from build123d import *

# Parameters (mm, degrees)
BOSS_EXTRUDE1_DEPTH      = 63.25
BOSS_EXTRUDE1_DEPTH_BACK = 63.25
CHAMFER1_SIZE            = 0.21


with BuildPart() as part:
    # Sketch3 → Boss-Extrude1 (new, two sides: drawn at the far end of the back side and taken through both)
    with BuildSketch(Plane.XY.offset(-BOSS_EXTRUDE1_DEPTH_BACK)):
        with BuildLine():
            Line((-2.5, 3.538348415), (-2.5, 6.538348415))
            ThreePointArc((-2.5, 6.538348415), (0, -7), (2.5, 6.538348415))
            Line((2.5, 6.538348415), (2.5, 3.538348415))
            Line((2.5, 3.538348415), (-2.5, 3.538348415))
        make_face()
    extrude(amount=BOSS_EXTRUDE1_DEPTH + BOSS_EXTRUDE1_DEPTH_BACK)

    # Chamfer1
    chamfer1_edges = [part.edges().sort_by_distance(p)[0] for p in [
        (0, -7, -63.25),
        (0, -7, 63.25),
    ]]
    chamfer(chamfer1_edges, length=CHAMFER1_SIZE)


solid = part.part
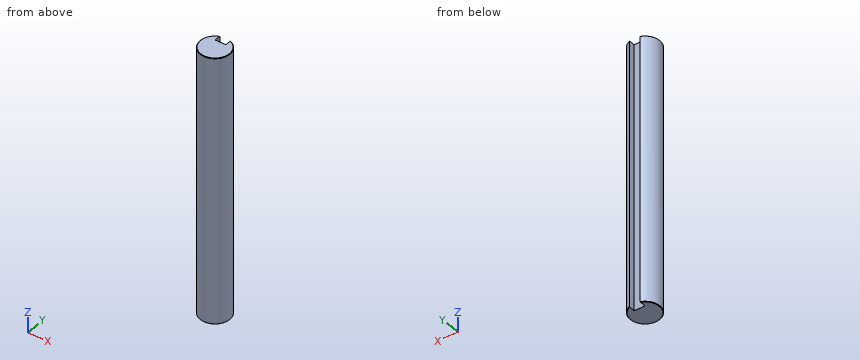
Could you check a few things on this model? Use its own coordinates, in mm. Give positions to 0.01 mm unless a question says otherwise; leave off trailing zeros. Write each loop counter-clockwise with the first axis right and the second up, starting at its lowest first coordinate (ties: lowest second). Pieces come first, ordered by that corner, then holes. Notation, with made-up numbers: (14, 80) -> (59, 80) arc R21 cw to (59, 113) -> close; hole circle Ø1 at (-32, 40). An arc over 180 degrees is marked (long way). Answer as CSV lines item,"result". Start each with the question number.
(1) If we section it at B-B, the plane x = 0: Write out the boundary of the cut face in (y, z), and give its area (3 significant figures).
(2) If we section it at A-A, the plane z = -0.5: Write out the boundary of the cut face in (x, y).
(3) Please list where these lines run through material, in increasing order: line 1 (X direction, y = 5.25, z = 34); line 2 (X direction, y = 4.25, z = 42); line 3 (Y direction, x = -0.25, z = 56).
(4) I'm going to push flat-ended pins straight in: pin 1 Ø2 at (x, z) = (4.5, -39) entering from -Y; pin 2 Ø0.9 at (y, z) = (4.5, 28) entering from -X; pin 3 Ø5 at (x, z) = (4.5, 29.5) entering from -Y. Where does each tip first touch, or does it pass through?
Answer list:
1,outline,"(-7, -63.04) -> (-6.79, -63.25) -> (3.54, -63.25) -> (3.54, 63.25) -> (-6.79, 63.25) -> (-7, 63.04) -> close"
1,area,"1,330 mm^2"
2,outline,"(-2.5, 3.54) -> (-2.5, 6.54) arc R7 ccw (long way) to (2.5, 6.54) -> (2.5, 3.54) -> close"
3,line 1,"-4.63 to -2.5, 2.5 to 4.63"
3,line 2,"-5.56 to -2.5, 2.5 to 5.56"
3,line 3,"-7 to 3.54"
4,pin 1,"y = -6.06"
4,pin 2,"x = -5.71"
4,pin 3,"y = -6.71"
